The figure shows three views and two pictorial views of one solid part (mm, origin at its lowest corner). Answer the questions. Give positions to 0.01 mm unless a question says otherwise; leave off trailing zeros. Order: outer loops, then holes, each group sorted by start corner. A loop starts at its lowest first (then second) coordinate and runs counter-clockwise, first axis right, second up. Notation, with made-up numbers: M 46.5,76.25 L 51.5,76.25 A15 cw 51.5,103.25 Z; hole C 21,56 d10. An arc over 180 degrees is marked long. One line per item, written item: value.
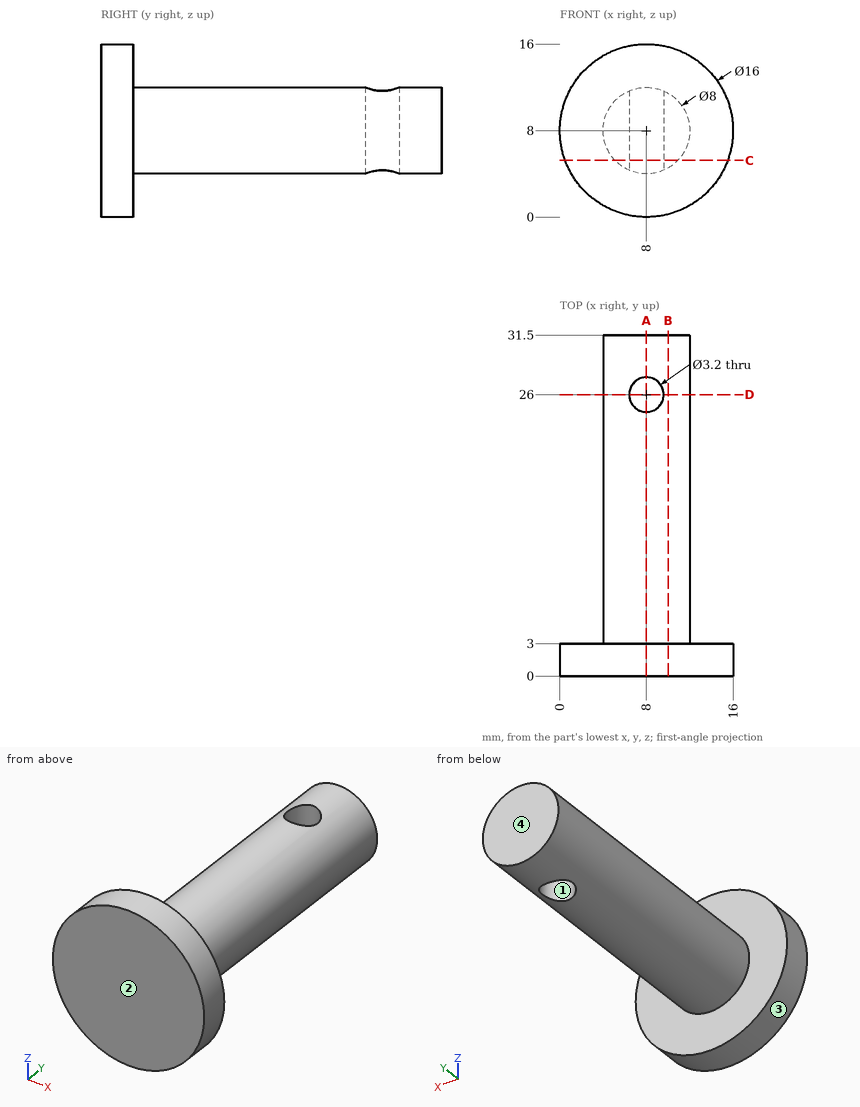
1) Find section C-C, the plane z = 5.25. Write down the section's boundary in (x, y).
Reported:
outline: M 0.49,0 L 15.51,0 L 15.51,3 L 10.9,3 L 10.9,31.5 L 5.1,31.5 L 5.1,3 L 0.49,3 Z; hole C 8,26 d3.2
2) Determine the mould class of the marked faces 1, 2, 3 and 4 for opening direction Y: +Y half, -Y half, draft (parallel to the pull), parting line (faces both ways), or undercut.
Reported:
face 1: undercut
face 2: -Y half
face 3: draft
face 4: +Y half
3) Find section A-A, the plane x = 8. Write down the section's boundary in (y, z).
Reported:
outline: M 0,0 L 3,0 L 3,4 L 24.4,4 L 24.4,12 L 3,12 L 3,16 L 0,16 Z; M 27.6,4 L 31.5,4 L 31.5,12 L 27.6,12 Z
4) Each of these flat-tipped pins is pushed along its axis until it touches: pin 1 Ø1 at (y, z) = (25.5, 4.5) entering from +X; pin 2 Ø1 at (x, y) = (11.5, 22) entering from -Z; pin 3 Ø2 at (y, z) = (22, 8) entering from -X. Where does it stop, or does it pass through?
Reported:
pin 1: stops at x = 10.65
pin 2: stops at z = 5.35
pin 3: stops at x = 4
5) Consider probe 1 along Y at (x, z) = (8, 6.5); probe 2 along X at (y, z) = (26, 10.25); probe 3 along Y at (x, z) = (2, 6). Determine where each line is inside the solid, lowest interval first.
Reported:
probe 1: y = 0 to 24.4, 27.6 to 31.5
probe 2: x = 4.69 to 6.4, 9.6 to 11.31
probe 3: y = 0 to 3
6) Find section D-D, the plane y = 26. Write down the section's boundary in (x, z), plus the area to 3 significant figures.
Reported:
outline: M 6.4,4.33 L 6.4,11.67 A4 ccw Z; M 9.6,4.33 A4 ccw 9.6,11.67 Z
area: 25.4 mm^2
7) Find section B-B, the plane x = 10. Write down the section's boundary in (y, z).
Reported:
outline: M 0,0.25 L 3,0.25 L 3,4.54 L 31.5,4.54 L 31.5,11.46 L 3,11.46 L 3,15.75 L 0,15.75 Z
